Input: part model. Units: mm. Frame: model coordinates. A direction names the side the tool comes from. Coordinates: 2 decimals unless noted, no trailing zeros. Loops run counter-clockwise (first coordinate to the right, second up) from the corner with the lowest first, then second, coordinate; pieces in that order, holes last.
Item 1: Ray query, line 1 along Z through (x, y) = (1, 14); line 2 along Y through (x, z) = (12, 32.5). Return the intervals inside material, ascending.
Item 2: Section D-D on z = 6.5. Return loops of the section in (x, y).
Item 3: Section B-B on z = 19. Return loops of the section in (x, y).
Item 4: Reachability of faces 5 (the flat face through (6, 8, 2)), 6 (the flat face through (27, 1, 12.1)), 7 (the cylindrical face through (1.014, 13.026, 10.852)) from +Z, -Z, +X, -X, +Y, -Y: full face, straight path, thin tool, end or side. Return the list, or none.
Item 5: Section A-A on x = 24. Return loops of the section in (y, z), and give its area (3 significant figures).
Item 6: Contact query for flat-ended pins moving along their axis: P1, Ø10, axis at y = 34, z = 36.5, coming from the +X side; P2, Ø6, axis at x = 9.5, z = 27.5, coming from the +Y side. Output: stop coordinate, or through.
Item 7: Pull-direction query (Z, two-part tool) for faces 1 (the cylindrical face through (10.355, 1.014, 39.976)), 2 (the flat face through (21, 0, 25)), 3 (the flat face through (9, 9, 0)), 4 (the cylindrical face through (1.01, 21.86, 32.47)); classes: released by +Z, released by -Z, zero draft, split by the parting line, or undercut.
Item 8: Section C-C on y = 20. Return loops of the section in (x, z).
```python
from build123d import *

# Parameters (mm, degrees)
BOSS_EXTRUDE1_DEPTH = 50
SKETCH2_R           = 11.05
SKETCH2_R_2         = 2
CUT_EXTRUDE1_DEPTH  = 88.761039192
CUT_EXTRUDE2_DEPTH  = 50
BOSS_EXTRUDE2_DEPTH = 2
BOSS_EXTRUDE3_DEPTH = 2
CHAMFER1_SIZE       = 5
SKETCH8_R           = 1.3611534
CUT_EXTRUDE3_DEPTH  = 10
SKETCH9_W           = 26.186270306
SKETCH9_H           = 50
CUT_EXTRUDE4_DEPTH  = 10


with BuildPart() as part:
    # Sketch1 → Boss-Extrude1 (new body)
    with BuildSketch(Plane.XY):
        Polygon((0, 0), (0, 51), (2, 51), (2, 2), (53, 2), (53, 0), align=None)
    extrude(amount=BOSS_EXTRUDE1_DEPTH)

    # Sketch2 → Cut-Extrude1 (cut, through all)
    with BuildSketch(Plane(origin=(2, 0, 0), x_dir=(0, 0, -1), z_dir=(1, 0, 0))):
        with Locations(Location((-25, 30, 0), (0, 0, 90))):
            Circle(SKETCH2_R)
        with Locations(Location((-40.5, 45.640445987, 0), (0, 0, 90))):
            Circle(SKETCH2_R_2)
        with Locations(Location((-9.5, 45.5, 0), (0, 0, 90))):
            Circle(SKETCH2_R_2)
        with Locations(Location((-40.5, 14.5, 0), (0, 0, 90))):
            Circle(SKETCH2_R_2)
        with Locations(Location((-9.5, 14.5, 0), (0, 0, 90))):
            Circle(SKETCH2_R_2)
    extrude(amount=-CUT_EXTRUDE1_DEPTH, mode=Mode.SUBTRACT)

    # Sketch3 → Cut-Extrude2 (cut)
    with BuildSketch(Plane(origin=(0, 2, 0), x_dir=(1, 0, 0), z_dir=(0, 1, 0))):
        with BuildLine():
            Line((12.455251015, -12.1), (42.544748985, -12.1))
            ThreePointArc((42.544748985, -12.1), (44.644629774, -9.977624237), (42.5, -7.900476833))
            Line((42.5, -7.900476833), (12.5, -7.900476833))
            ThreePointArc((12.5, -7.900476833), (10.355370226, -9.977624237), (12.455251015, -12.1))
        make_face()
        with BuildLine():
            Line((12.5, -42.099523167), (42.5, -42.099523167))
            ThreePointArc((42.5, -42.099523167), (44.644629774, -40.022375763), (42.544748985, -37.9))
            Line((42.544748985, -37.9), (12.455251015, -37.9))
            ThreePointArc((12.455251015, -37.9), (10.355370226, -40.022375763), (12.5, -42.099523167))
        make_face()
    extrude(amount=-CUT_EXTRUDE2_DEPTH, mode=Mode.SUBTRACT)

    # Sketch5 → Boss-Extrude2 (add)
    with BuildSketch(Plane.XY.offset(50)):
        Polygon((2, 22), (2, 4), (4, 2), (15, 2), align=None)
    extrude(amount=-BOSS_EXTRUDE2_DEPTH)

    # Sketch6 → Boss-Extrude3 (add)
    with BuildSketch(Plane(origin=(0, 0, 0), x_dir=(-1, 0, 0), z_dir=(0, 0, -1))):
        Polygon((-4, 2), (-2, 4), (-2, 22), (-15, 2), align=None)
    extrude(amount=-BOSS_EXTRUDE3_DEPTH)

    # Chamfer1
    chamfer1_edges = [part.edges().sort_by_distance(p)[0] for p in [
        (1, 51, 50),
        (1, 51, 0),
        (53, 1, 50),
        (53, 1, 0),
    ]]
    chamfer(chamfer1_edges, length=CHAMFER1_SIZE)

    # Sketch8 → Cut-Extrude3 (cut)
    with BuildSketch(Plane.ZY):
        with Locations(Location((35.606601718, 19.393398282, 0), (0, 0, 270))):
            Circle(SKETCH8_R)
        with Locations(Location((14.393398282, 19.393398282, 0), (0, 0, 270))):
            Circle(SKETCH8_R)
        with Locations(Location((14.393398282, 40.606601718, 0), (0, 0, 270))):
            Circle(SKETCH8_R)
        with Locations(Location((35.606601718, 40.606601718, 0), (0, 0, 270))):
            Circle(SKETCH8_R)
    extrude(amount=-CUT_EXTRUDE3_DEPTH, mode=Mode.SUBTRACT)

    # Sketch9 → Cut-Extrude4 (cut)
    with BuildSketch(Plane(origin=(0, 2, 0), x_dir=(1, 0, 0), z_dir=(0, 1, 0))):
        with Locations((55.093135153, -25)):
            Rectangle(SKETCH9_W, SKETCH9_H)
    extrude(amount=-CUT_EXTRUDE4_DEPTH, mode=Mode.SUBTRACT)


solid = part.part
```
Results found:
1. line 1: z = 0 to 7.56, 11.44 to 38.56, 42.44 to 50
1. line 2: y = 0 to 2
2. outline: (0, 0) - (42, 0) - (42, 2) - (2, 2) - (2, 51) - (0, 51) - close
3. outline: (0, 0) - (42, 0) - (42, 2) - (2, 2) - (2, 20.72) - (0, 20.72) - close; (0, 39.28) - (2, 39.28) - (2, 51) - (0, 51) - close
4. face 5: +X, +Y
4. face 6: +X, +Y, -Y
4. face 7: +X, -X
5. outline: (0, 0) - (2, 0) - (2, 7.9) - (0, 7.9) - close; (0, 12.1) - (2, 12.1) - (2, 37.9) - (0, 37.9) - close; (0, 42.1) - (2, 42.1) - (2, 50) - (0, 50) - close
5. area: 83.2 mm2
6. P1: stops at x = 2
6. P2: stops at y = 2
7. face 1: undercut
7. face 2: zero draft
7. face 3: released by -Z
7. face 4: undercut
8. outline: (0, 0) - (3.3, 0) - (3.3, 2) - (2, 2) - (2, 13.17) - (0, 13.17) - close; (0, 15.61) - (2, 15.61) - (2, 20.3) - (0, 20.3) - close; (0, 29.7) - (2, 29.7) - (2, 34.39) - (0, 34.39) - close; (0, 36.83) - (2, 36.83) - (2, 48) - (3.3, 48) - (3.3, 50) - (0, 50) - close
